Can you work these out from the model? Positions are in its coordinate system, mm. Face numbers are marked on the shaded views. A direction names the side the tool comes from. Coordinates: 2 decimals unless noted, no trailing zeros. Write each loop counter-clockwise with the first axis right and the second up, starting at its lowest first coordinate (ties: lowest second). Pieces come first, ordered by that corner, then holes.
```python
from build123d import *

# Parameters (mm, degrees)
F0_W     = 361.95
F0_H     = 285.75
F0_W_2   = 349.25
F0_H_2   = 273.05
F1_DEPTH = 88.9
F2_R     = 5.08
F4_D     = 25.4
F6_D     = 25.4


with BuildPart() as f1:
    # F0 (on Front) → F1 (new body, symmetric)
    with BuildSketch(Plane.XZ):
        Rectangle(F0_W, F0_H)
        Rectangle(F0_W_2, F0_H_2, mode=Mode.SUBTRACT)
    extrude(amount=F1_DEPTH, both=True)

    # F2
    f2_edges = [f1.edges().sort_by_distance(p)[0] for p in [
        (-174.625, 0, -136.525),
        (174.625, 0, -136.525),
        (174.625, 0, 136.525),
        (-174.625, 0, 136.525),
    ]]
    fillet(f2_edges, radius=F2_R)

    # F4 (through all)
    with Locations(Plane.XY.offset(142.875)):
        with Locations((-79.375005, 50.8), (79.375, 50.8)):
            Hole(F4_D / 2)

    # F6 (through all)
    with Locations(Plane(origin=(-180.975, 0, 0), x_dir=(0, -1, 0), z_dir=(-1, 0, 0))):
        with Locations((50.799999, 107.95), (50.8, -79.375006)):
            Hole(F6_D / 2)


solid = f1.part
```
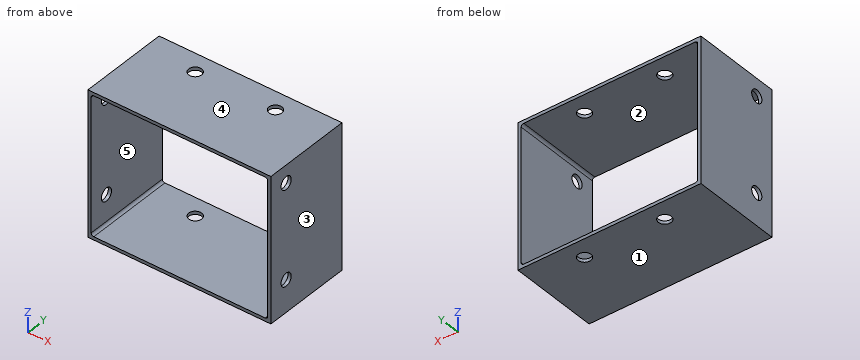
1. We'd pull the mould along X, two halves only. Please class the marked faces 1, 2 and 3: released by +X, released by -X, zero draft, split by the parting line, or undercut.
2. If we section it at A-A, the plane z = 18.5: List the corners of the cut face in (x, y) for me (3 decimals), plus the area to 3 significant figures.
3. If we section it at B-B, the plane y = 77: List the corners of the cut face in (x, z) for me (3 decimals).
4. Which directions (+Z, -Z, +X, -X, +Y, -Y) give clear straight access to the entire face, cutting with the end or side of a thin tool? Please do the marked faces 4 and 5.
5. If we section it at C-C, the plane z = 107.95: List the corners of the cut face in (x, y) for me (3 decimals).
6. If I drill on L1, parallel to Z at x = -177.25, y = -50.8 (3 decimals); L2, parallel to X at y = 50, z = -138 (3 decimals); L3, parallel to X at y = -68, z = -120 (3 decimals), over which ranges is the centre line in solid material (lowest first)?
7. If we section it at D-D, the plane x = 117: List the corners of the cut face in (y, z) for me (3 decimals), plus the area to 3 significant figures.
Answers:
1. face 1: zero draft
1. face 2: undercut
1. face 3: released by +X
2. outline: (-180.975, -88.9) - (-174.625, -88.9) - (-174.625, 88.9) - (-180.975, 88.9) - close; (174.625, -88.9) - (180.975, -88.9) - (180.975, 88.9) - (174.625, 88.9) - close
2. area: 2,260 mm2
3. outline: (-180.975, -142.875) - (180.975, -142.875) - (180.975, 142.875) - (-180.975, 142.875) - close; hole (-174.625, -131.445) arc R5.08 ccw to (-169.545, -136.525) - (169.545, -136.525) arc R5.08 ccw to (174.625, -131.445) - (174.625, 131.445) arc R5.08 ccw to (169.545, 136.525) - (-169.545, 136.525) arc R5.08 ccw to (-174.625, 131.445) - close
4. face 4: +Z, +X, -X, +Y, -Y
4. face 5: +Y, -Y
5. outline: (-180.975, -88.9) - (-174.625, -88.9) - (-174.625, -63.5) - (-180.975, -63.5) - close; (-180.975, -38.1) - (-174.625, -38.1) - (-174.625, 88.9) - (-180.975, 88.9) - close; (174.625, -88.9) - (180.975, -88.9) - (180.975, -63.5) - (174.625, -63.5) - close; (174.625, -38.1) - (180.975, -38.1) - (180.975, 88.9) - (174.625, 88.9) - close
6. L1: z = -142.875 to -92.075, -66.675 to 95.25, 120.65 to 142.875
6. L2: x = -180.975 to -92.05, -66.7 to 66.7, 92.05 to 180.975
6. L3: x = -180.975 to -174.625, 174.625 to 180.975
7. outline: (-88.9, -142.875) - (88.9, -142.875) - (88.9, -136.525) - (-88.9, -136.525) - close; (-88.9, 136.525) - (88.9, 136.525) - (88.9, 142.875) - (-88.9, 142.875) - close
7. area: 2,260 mm2
